from build123d import *

# Parameters (mm, degrees)
SKETCH1_R           = 65.3
SKETCH1_R_2         = 45.3
SKETCH1_R_3         = 1.65
BOSS_EXTRUDE1_DEPTH = 10
FILLET1_R           = 5


with BuildPart() as part:
    # Sketch1 → Boss-Extrude1 (new body)
    with BuildSketch(Plane.XY):
        Circle(SKETCH1_R)
        Circle(SKETCH1_R_2, mode=Mode.SUBTRACT)
        with Locations((35.461405077, -35.461405077)):
            Circle(SKETCH1_R_3, mode=Mode.SUBTRACT)
        with Locations((0, -50.15)):
            Circle(SKETCH1_R_3, mode=Mode.SUBTRACT)
        with Locations((-35.461405077, -35.461405077)):
            Circle(SKETCH1_R_3, mode=Mode.SUBTRACT)
        with Locations((-50.15, 0)):
            Circle(SKETCH1_R_3, mode=Mode.SUBTRACT)
        with Locations((-35.461405077, 35.461405077)):
            Circle(SKETCH1_R_3, mode=Mode.SUBTRACT)
        with Locations((0, 50.15)):
            Circle(SKETCH1_R_3, mode=Mode.SUBTRACT)
        with Locations((35.461405077, 35.461405077)):
            Circle(SKETCH1_R_3, mode=Mode.SUBTRACT)
        with Locations((50.15, 0)):
            Circle(SKETCH1_R_3, mode=Mode.SUBTRACT)
    extrude(amount=BOSS_EXTRUDE1_DEPTH)

    # Fillet1
    fillet1_edges = [part.edges().sort_by_distance(p)[0] for p in [
        (-65.3, 0, 10),
    ]]
    fillet(fillet1_edges, radius=FILLET1_R)


solid = part.part
Check sheet for the modelled part. Datum: model origin and axes. Units: mm. Round coordinates to 2 decimals unless told otherwise and drop trailing zeros. Order: outer loops, then holes, each group sorted by start corner. A loop starts at its lowest first (then second) coordinate and runs counter-clockwise, first axis right, second up.
(1) Go/stop test with flat-tipped pins: P1, Ø5, axis at x = 47, z = 7, coming from the +Y side; P2, Ø2, axis at y = -47.5, z = 1.5, coming from the +X side; P3, Ø2, axis at x = -29.5, z = 7.5, coming from the +Y side. Record where each tip stops, or that it passes through.
(2) Cross-section at A-A, the plane x = 0. Enter the section's corners in (y, z), and give its area (3 significant figures).
(3) Scan lines: probe 1 along Y at (x, z) = (1, 7.75); probe 2 along Y at (x, z) = (6.5, 5.5); probe 3 along X at (y, z) = (22.5, 9.25). Record each from-to range of solid material in increasing order.
(4) Cross-section at B-B, the plane z = 7.5. State how many separate pieces and enclosed holes the cut face has, and give its area (3 significant figures).
(5) Draft check along Y on faces 1 (the flat face through (-15, -43, 0)), 2 (the cylindrical face through (62.285, 19.614, 2.465)), 3 (the cylindrical face through (-37.11, -35.39, 4.93)). Enter one of: pulls with the +Y half, pulls with the -Y half, needs draft (parallel to the pull), parting line crosses it, or undercut.
Check sheet entries:
1. P1: stops at y = 47.47
1. P2: stops at x = 45.85
1. P3: stops at y = 58.24
2. outline: (-65.3, 0) - (-51.8, 0) - (-51.8, 10) - (-60.3, 10) arc R5 ccw to (-65.3, 5) - close; (-48.5, 0) - (-45.3, 0) - (-45.3, 10) - (-48.5, 10) - close; (45.3, 0) - (48.5, 0) - (48.5, 10) - (45.3, 10) - close; (51.8, 0) - (65.3, 0) - (65.3, 5) arc R5 ccw to (60.3, 10) - (51.8, 10) - close
2. area: 323 mm2
3. probe 1: y = -64.47 to -51.46, -48.84 to -45.29, 45.29 to 48.84, 51.46 to 64.47
3. probe 2: y = -64.95 to -44.83, 44.83 to 64.95
3. probe 3: x = -58.77 to -39.32, 39.32 to 58.77
4. separate pieces: 1
4. enclosed holes: 9
4. area: 6,610 mm2
5. face 1: needs draft
5. face 2: parting line crosses it
5. face 3: undercut
